For this review, take the finished solid that the model builds, in its own axes (mm). A direction names the side the tool comes from. Coordinates: 2 decimals unless noted, no trailing zeros. Loops run counter-clockwise (first coordinate to the right, second up) from the corner with the lowest first, then second, coordinate; pieces in that order, holes last. Notation, with made-up numbers: M -19.5,-11.75 L -10.5,-11.75 A4 cw -10.5,-4.75 Z; hole C -23.75,73 d5. An arc over 180 degrees is marked long. Put each result on its own line as item: value.
```python
from build123d import *

# Parameters (mm, degrees)
SKETCH1_W           = 20.5
SKETCH1_H           = 60.5
SKETCH1_R           = 2.45
BOSS_EXTRUDE1_DEPTH = 3
SKETCH2_W           = 26.5
SKETCH2_H           = 66.5
SKETCH2_W_2         = 20.5
SKETCH2_H_2         = 60.5
BOSS_EXTRUDE2_DEPTH = 6


with BuildPart() as part:
    # Sketch1 → Boss-Extrude1 (new body)
    with BuildSketch(Plane(origin=(0, 0, 0), x_dir=(1, 0, 0), z_dir=(0, 1, 0))):
        with Locations((10.25, 30.25)):
            Rectangle(SKETCH1_W, SKETCH1_H)
        with Locations(Location((10.25, 10.25, 0), (0, 0, 270))):
            Circle(SKETCH1_R, mode=Mode.SUBTRACT)
        with Locations(Location((10.25, 50.25, 0), (0, 0, 270))):
            Circle(SKETCH1_R, mode=Mode.SUBTRACT)
        with Locations(Location((10.25, 30.25, 0), (0, 0, 270))):
            Circle(SKETCH1_R, mode=Mode.SUBTRACT)
    extrude(amount=BOSS_EXTRUDE1_DEPTH)

    # Sketch2 → Boss-Extrude2 (add)
    with BuildSketch(Plane(origin=(0, 3, 0), x_dir=(1, 0, 0), z_dir=(0, 1, 0))):
        with Locations((10.25, 30.25)):
            Rectangle(SKETCH2_W, SKETCH2_H)
        with Locations((10.25, 30.25)):
            Rectangle(SKETCH2_W_2, SKETCH2_H_2, mode=Mode.SUBTRACT)
    extrude(amount=-BOSS_EXTRUDE2_DEPTH)


solid = part.part
```
(1) Add section B-B (y = -2.35). Write out the cut boundary in (x, z), plus the area to 3 significant figures.
Determined:
outline: M -3,-63.5 L 23.5,-63.5 L 23.5,3 L -3,3 Z; hole M 0,-60.5 L 20.5,-60.5 L 20.5,0 L 0,0 Z
area: 522 mm^2
(2) Add section C-C (x = 10.25). Write out the cut boundary in (y, z).
Determined:
outline: M -3,-63.5 L 3,-63.5 L 3,-52.7 L 0,-52.7 L 0,-60.5 L -3,-60.5 Z; M -3,0 L 0,0 L 0,-7.8 L 3,-7.8 L 3,3 L -3,3 Z; M 0,-47.8 L 3,-47.8 L 3,-32.7 L 0,-32.7 Z; M 0,-27.8 L 3,-27.8 L 3,-12.7 L 0,-12.7 Z
(3) For pin 1 (6.5 mm diameter, centred on x = 10.25, z = -30.25, fed in from -Y); pin 2 (5 mm diameter, centred on x = 19.5, z = -22.5, fed in from -Y), all flat-tipped, find the tip position at first contact; note any pin that passes through.
Determined:
pin 1: stops at y = 0
pin 2: stops at y = -3
(4) Add section A-A (z = -10.25). Write out the cut boundary in (x, y).
Determined:
outline: M -3,-3 L 0,-3 L 0,0 L 7.8,0 L 7.8,3 L -3,3 Z; M 12.7,0 L 20.5,0 L 20.5,-3 L 23.5,-3 L 23.5,3 L 12.7,3 Z
(5) Add section D-D (y = 1.45). Write out the cut boundary in (x, z).
Determined:
outline: M -3,-63.5 L 23.5,-63.5 L 23.5,3 L -3,3 Z; hole C 10.25,-50.25 d4.9; hole C 10.25,-30.25 d4.9; hole C 10.25,-10.25 d4.9
(6) Wall thickness on line 1 along Z through (x, y) = (11.5, -1.3); line 2 along X through (y, z) = (0.9, -30.25); line 3 along X through (y, z) = (-1.65, -11): over which ranges is each line inside the solid? List them lowest first. Write a range as [from, to].
Determined:
line 1: z = [-63.5, -60.5], [0, 3]
line 2: x = [-3, 7.8], [12.7, 23.5]
line 3: x = [-3, 0], [20.5, 23.5]
(7) Tool access review of faces 5 (the flat face through (7, 3, -31)), 6 (the flat face through (6, 0, -31)): name each direction out of +Z, -Z, +X, -X, +Y, -Y from which nothing blocks a thin tool from reaching the whole face with its end or side.
Determined:
face 5: +Z, -Z, +X, -X, +Y
face 6: -Y
(8) Draft analysis for pull direction Z (two halves, no side actions). For faces 1 (the flat face through (10, 0, 3)), 2 (the flat face through (10, 0, -63.5)), 3 (the flat face through (-3, 0, -30)), 4 (the flat face through (10, -1, 0)), state which applies: +Z half, -Z half, draft (parallel to the pull), parting line (faces both ways), or undercut.
Determined:
face 1: +Z half
face 2: -Z half
face 3: draft
face 4: undercut
